CAD build for the part. Positions are in the model's coordinates, mm. A direction names the side the tool comes from. Give positions to 0.01 mm unless a question says otherwise; leave off trailing zeros. Loops run counter-clockwise (first coordinate to the right, second up) from the corner with the lowest first, then second, coordinate; pieces in that order, holes last.
```python
from build123d import *

# Parameters (mm, degrees)
F0_R     = 7.5
F0_R_2   = 4
F1_DEPTH = 18
F2_R     = 6.5
F2_R_2   = 4
F3_DEPTH = 9
F4_SIZE  = 1
F5_SIZE  = 0.5
F6_R     = 9.5
F6_R_2   = 6.5
F7_DEPTH = 2
F8_R     = 2
F9_DEPTH = 25


with BuildPart() as f1:
    # F0 (on Top) → F1 (new body)
    with BuildSketch(Plane.XY):
        Circle(F0_R)
        Circle(F0_R_2, mode=Mode.SUBTRACT)
    extrude(amount=F1_DEPTH)

    # F2 (on face) → F3 (join)
    with BuildSketch(Plane.XY.offset(18)):
        Circle(F2_R)
        Circle(F2_R_2, mode=Mode.SUBTRACT)
    extrude(amount=F3_DEPTH)

    # F4
    f4_edges = [f1.edges().sort_by_distance(p)[0] for p in [
        (-4, 0, 27),
        (-4, 0, 0),
    ]]
    chamfer(f4_edges, length=F4_SIZE)

    # F5
    f5_edges = [f1.edges().sort_by_distance(p)[0] for p in [
        (-7.5, 0, 0),
        (-6.5, 0, 27),
    ]]
    chamfer(f5_edges, length=F5_SIZE)

    # F6 (on face) → F7 (join)
    with BuildSketch(Plane.XY.offset(18)):
        Circle(F6_R)
        Circle(F6_R_2, mode=Mode.SUBTRACT)
    extrude(amount=-F7_DEPTH)

    # F8 (on Front) → F9 (cut)
    with BuildSketch(Plane.XZ):
        with Locations((0, 5)):
            Circle(F8_R)
        with Locations((0, 12)):
            Circle(F8_R)
    extrude(amount=F9_DEPTH, mode=Mode.SUBTRACT)


solid = f1.part
```
1. Tool access for faces 1 (the face through (-4, 4, 27)), 2 (the face through (1.847, -5.458, 11.234)), 3 (the face through (-0.976, 7.436, 8.142)), 4 (the face through (4, -6, 18)): list every direction of +Z, -Z, +X, -X, +Y, -Y with a clear straight run to the whole face (end or side of a thin tool).
Responses:
face 1: +Z, +X, -X, +Y, -Y
face 2: -Y
face 3: -Z
face 4: +Z
2. Drop flat-ended pins along their axis: pin 1 (1.5 mm diameter, centred on x = -0.5, y = -1.5, fed in from +Z); pin 2 (5 mm diameter, centred on y = -2.5, z = 7.5, fed in from +X); pin 3 (6.5 mm diameter, centred on x = 0, z = 12, fed in from -Y); pin 4 (4 mm diameter, centred on x = 1.5, z = 22, fed in from -Y). Give the stop position or say it passes through.
Responses:
pin 1: passes through
pin 2: stops at x = 7.5
pin 3: stops at y = -7.5
pin 4: stops at y = -6.5
3. Probe line 1 along Z through (x, y) = (0, -6); line 2 along Y through (x, z) = (0, 14.75); line 3 along Z through (x, y) = (2.5, -8.25). List the from-to ranges inside material, lowest first.
Responses:
line 1: z = 0 to 3, 7 to 10, 14 to 27
line 2: y = -7.5 to -4, 4 to 7.5
line 3: z = 16 to 18
4. Saw through at D-D, the plane z = 8.75. List the corners of the cut face in (x, y), and give its area (3 significant figures).
Responses:
outline: circle Ø15 at (0, 0); hole circle Ø8 at (0, 0)
area: 126 mm2
5. Saw through at B-B, the plane y = 0. List the corners of the cut face in (x, z).
Responses:
outline: (-9.5, 16) - (-7.5, 16) - (-7.5, 0.5) - (-7, 0) - (-5, 0) - (-4, 1) - (-4, 26) - (-5, 27) - (-6, 27) - (-6.5, 26.5) - (-6.5, 18) - (-9.5, 18) - close; (4, 1) - (5, 0) - (7, 0) - (7.5, 0.5) - (7.5, 16) - (9.5, 16) - (9.5, 18) - (6.5, 18) - (6.5, 26.5) - (6, 27) - (5, 27) - (4, 26) - close
6. Pull direction X, two halves, no side cores. Call faces 5 (the face through (-5.158, -3.955, 22.19)), 6 (the face through (1.847, -5.458, 4.234)), 7 (the face through (1, 8, 16)): released by +X, released by -X, zero draft, split by the parting line, or undercut.
Responses:
face 5: split by the parting line
face 6: undercut
face 7: zero draft
7. Saw through at C-C, the plane z = 16.5. List the corners of the cut face in (x, y), and give its area (3 significant figures).
Responses:
outline: circle Ø19 at (0, 0); hole circle Ø8 at (0, 0)
area: 233 mm2
8. Saw through at A-A, the plane x = 0. Count the separate pieces of the cut face and the enclosed holes in it, and give its area (4 significant figures).
Responses:
separate pieces: 4
enclosed holes: 0
area: 148.5 mm2
